The model under review builds one solid part; all positions refer to its coordinate system, in mm. A direction names the side the tool comes from. Give positions to 0.01 mm unless a question says otherwise; leave off trailing zeros. Write each loop counter-clockwise with the first axis right and the second up, starting at its lowest first coordinate (ties: lowest second). Pieces come first, ordered by that corner, then holes. Notation, with made-up numbers: (-14, -2.75) - (44, -2.75) arc R22 cw to (44, 35.25) - close; hole circle Ø11 at (77.25, 9.5). An arc over 180 degrees is marked (long way). Write item = value, one per line.
```python
from build123d import *

# Parameters (mm, degrees)
SKETCH_1_W          = 29
SKETCH_1_H          = 29
EXTRUDE_1_DEPTH     = 32.7
SKETCH_2_R          = 14.5
SKETCH_2_R_2        = 12.995867769
EXTRUDE_2_DEPTH     = 7.4
SKETCH_3_R          = 1.5
CUT_EXTRUDE_1_DEPTH = 42.4
SKETCH_4_R          = 18
EXTRUDE_3_DEPTH     = 32.9


with BuildPart() as part:
    # 草图1 → 凸台-拉伸1 (new body)
    with BuildSketch(Plane.XY):
        Rectangle(SKETCH_1_W, SKETCH_1_H)
    extrude(amount=EXTRUDE_1_DEPTH)

    # 草图2 → 凸台-拉伸2 (add)
    with BuildSketch(Plane.XY.offset(32.7)):
        Circle(SKETCH_2_R)
        Circle(SKETCH_2_R_2, mode=Mode.SUBTRACT)
    extrude(amount=EXTRUDE_2_DEPTH)

    # 草图3 → 切除-拉伸1 (cut)
    with BuildSketch(Plane.ZY.offset(14.5)):
        with Locations(Location((2, 10, 0), (0, 0, 270))):
            Circle(SKETCH_3_R)
        with Locations(Location((30.7, 10, 0), (0, 0, 270))):
            Circle(SKETCH_3_R)
        with Locations(Location((30.7, -10, 0), (0, 0, 270))):
            Circle(SKETCH_3_R)
        with Locations(Location((2, -10, 0), (0, 0, 270))):
            Circle(SKETCH_3_R)
    extrude(amount=-CUT_EXTRUDE_1_DEPTH, mode=Mode.SUBTRACT)

    # 草图4 → 凸台-拉伸3 (add)
    with BuildSketch(Plane.XY.offset(40.1)):
        Circle(SKETCH_4_R)
    extrude(amount=EXTRUDE_3_DEPTH)


solid = part.part
```
1. Machinability: for faces 4 (the flat face through (11, 12, 32.7)), 5 (the cylindrical face through (-2.343, 17.847, 56.32)), 6 (the flat face through (-14.5, 0, 16)), 7 (the flat face through (-12, -11, 32.7)), 8 (the flat face through (0, 0, 32.7)), which of the approach directions +Z, -Z, +X, -X, +Y, -Y give a long, thin tool a straight path to every point of the face, cutting with its end or side? Answer none if there is none.
Findings below:
face_4 = +X, +Y
face_5 = +Z
face_6 = -Z, -X, +Y, -Y
face_7 = -X, -Y
face_8 = none
2. Take a section at B-B on x = -3. Give the boundary of the cut face in (y, z).
Findings below:
outline = (-17.75, 40.1) - (-14.19, 40.1) - (-14.19, 32.7) - (-14.5, 32.7) - (-14.5, 0) - (14.5, 0) - (14.5, 32.7) - (14.19, 32.7) - (14.19, 40.1) - (17.75, 40.1) - (17.75, 73) - (-17.75, 73) - close; hole (-12.64, 32.7) - (12.64, 32.7) - (12.64, 40.1) - (-12.64, 40.1) - close; hole circle Ø3 at (-10, 2); hole circle Ø3 at (-10, 30.7); hole circle Ø3 at (10, 2); hole circle Ø3 at (10, 30.7)
3. For line 1 (Z direction, x = 8, y = -10); line 2 (Z direction, x = 10, y = -0.5); line 3 (Z direction, x = -7.5, y = 9), list the stretches that pass through material, from the lowest coordinate up. Write a range as from..to.
Findings below:
line_1 = 0..0.5, 3.5..29.2, 32.2..32.7, 40.1..73
line_2 = 0..32.7, 40.1..73
line_3 = 0..0.88, 3.12..29.58, 31.82..32.7, 40.1..73
4. Take a section at C-C on y = -4. Give the boundary of the cut face in (x, z), and give its area (3 significant figures).
Findings below:
outline = (-17.55, 40.1) - (-13.94, 40.1) - (-13.94, 32.7) - (-14.5, 32.7) - (-14.5, 0) - (14.5, 0) - (14.5, 32.7) - (13.94, 32.7) - (13.94, 40.1) - (17.55, 40.1) - (17.55, 73) - (-17.55, 73) - close; hole (-12.36, 32.7) - (12.36, 32.7) - (12.36, 40.1) - (-12.36, 40.1) - close
area = 2,130 mm²
5. Take a section at D-D on z = 49. Give the boundary of the cut face in (x, y).
Findings below:
outline = circle Ø36 at (0, 0)
6. Draft analysis for pull direction Z (two halves, no side actions). For faces 1 (the flat face through (0, -14.5, 16)), 2 (the flat face through (1, 15, 40.1)), 3 (the flat face through (0, 0, 73)), state which applies: +Z half, -Z half, draft (parallel to the pull), parting line (faces both ways), or undercut.
Findings below:
face_1 = draft
face_2 = undercut
face_3 = +Z half
7. Insertion check: P1, Ø5, axis at x = 12, z = 51, coming from the -Y side; P2, Ø8.5, axis at y = -5.5, z = 9, coming from the -X side; P3, Ø14.5, axis at y = 0.5, z = 10.5, coming from the +X side; P4, Ø2.5, axis at y = 10, z = 30.7, coming from the +X side. Each pin has a flat end and moves straight along its axis. Give the tip position at first contact, or say it passes through.
Findings below:
P1 = -15.29
P2 = -14.5
P3 = 14.5
P4 = through
8. Take a section at A-A on y = 9.5. Give the boundary of the cut face in (x, z).
Findings below:
outline = (-15.29, 40.1) - (-10.95, 40.1) - (-10.95, 32.7) - (-14.5, 32.7) - (-14.5, 32.11) - (14.5, 32.11) - (14.5, 32.7) - (10.95, 32.7) - (10.95, 40.1) - (15.29, 40.1) - (15.29, 73) - (-15.29, 73) - close; (-14.5, 0) - (14.5, 0) - (14.5, 0.59) - (-14.5, 0.59) - close; (-14.5, 3.41) - (14.5, 3.41) - (14.5, 29.29) - (-14.5, 29.29) - close; hole (-8.87, 32.7) - (8.87, 32.7) - (8.87, 40.1) - (-8.87, 40.1) - close
